Design review of the part shown in the three views and the two pictorial views. Dimensions are in mm from the part's minimum x, y and z. Give positions to 0.01 mm unless a question says otherwise; leave off trailing zeros. Loops run counter-clockwise (first coordinate to the right, second up) from the corner with the lowest first, then second, coordinate; pieces in that order, holes last. Notation, with made-up numbers: (88.25, -34.5) -> (134.25, -34.5) arc R19 cw to (134.25, -15.5) -> close; hole circle Ø10 at (29.25, 64.25). An arc over 180 degrees is marked (long way). Answer as CSV lines item,"result".
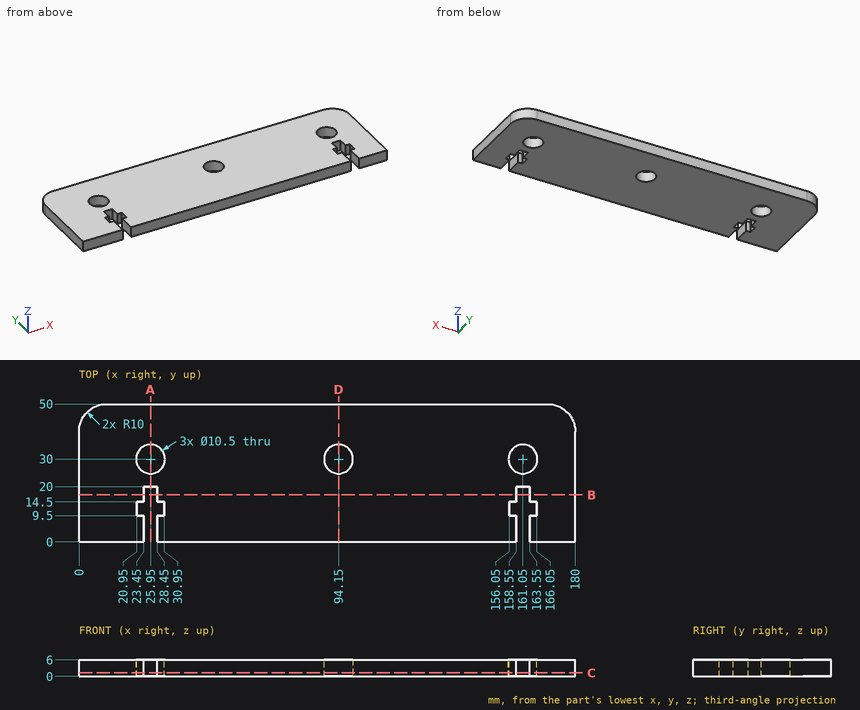
Q1. We need section D-D, the plane x = 94.15. State the section outline as (y, z) points, and give its area (3 significant figures).
Filled sheet:
outline,"(0, 0) -> (24.75, 0) -> (24.75, 6) -> (0, 6) -> close; (35.25, 0) -> (50, 0) -> (50, 6) -> (35.25, 6) -> close"
area,"237 mm^2"
Q2. We need section A-A, the plane x = 25.95. State the section outline as (y, z) points.
Filled sheet:
outline,"(20, 0) -> (24.75, 0) -> (24.75, 6) -> (20, 6) -> close; (35.25, 0) -> (50, 0) -> (50, 6) -> (35.25, 6) -> close"
Q3. Clearance check with a flat-ended pin moving along its axis: pin 1 Ø8.5 at (x, y) = (25.95, 30) entering from +Z. State where the tip first meets the part, or that it passes through.
Filled sheet:
pin 1,"passes through"
Q4. We need section C-C, the plane z = 1.3. State how many separate pieces and enclosed holes the cut face has, and give its area (3 significant figures).
Filled sheet:
separate pieces,"1"
enclosed holes,"3"
area,"8,450 mm^2"
Q5. We need section B-B, the plane y = 17. State the section outline as (x, z) points.
Filled sheet:
outline,"(0, 0) -> (23.45, 0) -> (23.45, 6) -> (0, 6) -> close; (28.45, 0) -> (158.55, 0) -> (158.55, 6) -> (28.45, 6) -> close; (163.55, 0) -> (180, 0) -> (180, 6) -> (163.55, 6) -> close"
Q6. To check wall thickness, follow probe 1 along X at (y, z) = (16, 1.25); probe 2 along Y at (x, z) = (161.05, 3.5); probe 3 along X at (y, z) = (28, 3.25). State the ranges of each line that lie inside material, in increasing order. Write a range as from..to.
Filled sheet:
probe 1,"x = 0..23.45, 28.45..158.55, 163.55..180"
probe 2,"y = 20..24.75, 35.25..50"
probe 3,"x = 0..21.1, 30.8..89.3, 99..156.2, 165.9..180"
